Check sheet for the modelled part. Datum: model origin and axes. Units: mm. A direction names the side the tool comes from. Round coordinates to 2 decimals unless told otherwise and drop trailing zeros. Loops run counter-clockwise (first coordinate to the right, second up) from the corner with the lowest first, then second, coordinate; pieces in that order, holes last. Notation, with made-up numbers: M 19.25,23.5 L 76.25,23.5 A32 cw 76.25,57.5 Z; hole C 0.5,-36 d11. An arc over 180 degrees is marked long. Write item = value, one per line. Start each with the question number.
(1) Mould release check, pull along X, two halves, no side actions. Record for faces 5 (the face through (-22.944, 19, 4)), 6 (the face through (-13.641, 19, 4)), 7 (the face through (0, -25.5, 1)), 8 (the face through (-6.5, 3, 3)): pulls with the +X half, pulls with the -X half, needs draft (parallel to the pull), parting line crosses it, or undercut.
(2) Cross-section at C-C on y = 4.5. Record the boundary of the cut face in (x, z).
(3) Scan lines: L1, parallel to X at y = -7, z = 3.2; L2, parallel to Z at x = 19.5, y = 13; L3, parallel to X at y = 13, z = 2.8. Record each from-to range of solid material in increasing order. Write a range as from..to.
(4) Cross-section at D-D on x = 9. Record the boundary of the cut face in (y, z).
(5) Cross-section at B-B on x = -16.5. Record the boundary of the cut face in (y, z).
(6) Set-up check for faces 1 (the face through (7, -10.5, 3)), 2 (the face through (-22.944, -5, 4)), 3 (the face through (-19, -15.641, 4)), 4 (the face through (-19, -20.252, 4)): record each of +Z, -Z, +X, -X, +Y, -Y from which the full face is reachable in a straight line by a thin tool's end or side.
(7) Go/stop test with flat-tipped pins: P1, Ø22.5, axis at x = 5.5, y = -3, coming from the +Z side; P2, Ø1.3, axis at x = -20.5, z = 4, coming from the -Y side; P3, Ø2, axis at y = -5.5, z = 5, coming from the -X side. Record where each tip stops, or that it passes through.
(8) Cross-section at A-A on z = 3.15. Record the boundary of the cut face in (x, y), plus the area to 3 significant figures.
from build123d import *

# Parameters (mm, degrees)
SKETCH1_W           = 51
SKETCH1_H           = 51
SKETCH1_W_2         = 28
SKETCH1_H_2         = 28
SKETCH1_W_3         = 9.30278776
SKETCH1_H_3         = 12.209946987
SKETCH1_W_4         = 8.24332
SKETCH1_H_4         = 4.56356538
SKETCH1_H_5         = 4.61067604
BOSS_EXTRUDE1_DEPTH = 1.5748
SKETCH1_2_W         = 28
SKETCH1_2_H         = 28
BOSS_EXTRUDE2_DEPTH = 4
SKETCH1_3_W         = 9.30278776
SKETCH1_3_H         = 12.209946987
SKETCH1_3_W_2       = 8.24332
SKETCH1_3_H_2       = 4.56356538
SKETCH1_3_H_3       = 4.61067604
BOSS_EXTRUDE3_DEPTH = 6


with BuildPart() as part:
    # Sketch1 → Boss-Extrude1 (new body)
    with BuildSketch(Plane.XY):
        Rectangle(SKETCH1_W, SKETCH1_H)
        with Locations((7.5, 3.5)):
            Rectangle(SKETCH1_W_2, SKETCH1_H_2, mode=Mode.SUBTRACT)
        with Locations((-18.29281594, 18.874000471)):
            Rectangle(SKETCH1_W_3, SKETCH1_H_3, mode=Mode.SUBTRACT)
        with Locations((-18.82254982, -4.74850311)):
            Rectangle(SKETCH1_W_4, SKETCH1_H_4, mode=Mode.SUBTRACT)
        with Locations((-18.82254982, -11.33562382)):
            Rectangle(SKETCH1_W_4, SKETCH1_H_5, mode=Mode.SUBTRACT)
        with Locations((-18.82254982, -17.94629986)):
            Rectangle(SKETCH1_W_4, SKETCH1_H_5, mode=Mode.SUBTRACT)
    extrude(amount=BOSS_EXTRUDE1_DEPTH)

    # Sketch1<2> → Boss-Extrude2 (add)
    with BuildSketch(Plane.XY):
        with Locations((7.5, 3.5)):
            Rectangle(SKETCH1_2_W, SKETCH1_2_H)
    extrude(amount=BOSS_EXTRUDE2_DEPTH)

    # Sketch1<3> → Boss-Extrude3 (add)
    with BuildSketch(Plane.XY):
        with Locations((-18.29281594, 18.874000471)):
            Rectangle(SKETCH1_3_W, SKETCH1_3_H)
        with Locations((-18.82254982, -4.74850311)):
            Rectangle(SKETCH1_3_W_2, SKETCH1_3_H_2)
        with Locations((-18.82254982, -11.33562382)):
            Rectangle(SKETCH1_3_W_2, SKETCH1_3_H_3)
        with Locations((-18.82254982, -17.94629986)):
            Rectangle(SKETCH1_3_W_2, SKETCH1_3_H_3)
    extrude(amount=BOSS_EXTRUDE3_DEPTH)


solid = part.part
Result:
q1.face_5 = pulls with the -X half
q1.face_6 = undercut
q1.face_7 = needs draft
q1.face_8 = undercut
q2.outline = M -25.5,0 L 25.5,0 L 25.5,1.57 L 21.5,1.57 L 21.5,4 L -6.5,4 L -6.5,1.57 L -25.5,1.57 Z
q3.L1 = -22.94..-14.7, -6.5..21.5
q3.L2 = 0..4
q3.L3 = -22.94..-13.64, -6.5..21.5
q4.outline = M -25.5,0 L 25.5,0 L 25.5,1.57 L 17.5,1.57 L 17.5,4 L -10.5,4 L -10.5,1.57 L -25.5,1.57 Z
q5.outline = M -25.5,0 L 25.5,0 L 25.5,1.57 L 24.98,1.57 L 24.98,6 L 12.77,6 L 12.77,1.57 L -2.47,1.57 L -2.47,6 L -7.03,6 L -7.03,1.57 L -9.03,1.57 L -9.03,6 L -13.64,6 L -13.64,1.57 L -15.64,1.57 L -15.64,6 L -20.25,6 L -20.25,1.57 L -25.5,1.57 Z
q6.face_1 = +Z, +X, -Y
q6.face_2 = +Z, -X, +Y, -Y
q6.face_3 = +Z, +X, -X
q6.face_4 = +Z, +X, -X, -Y
q7.P1 = 4
q7.P2 = -20.25
q7.P3 = -22.94
q8.outline = M -22.94,-20.25 L -14.7,-20.25 L -14.7,-15.64 L -22.94,-15.64 Z; M -22.94,-13.64 L -14.7,-13.64 L -14.7,-9.03 L -22.94,-9.03 Z; M -22.94,-7.03 L -14.7,-7.03 L -14.7,-2.47 L -22.94,-2.47 Z; M -22.94,12.77 L -13.64,12.77 L -13.64,24.98 L -22.94,24.98 Z; M -6.5,-10.5 L 21.5,-10.5 L 21.5,17.5 L -6.5,17.5 Z
q8.area = 1,010 mm^2
